Design review of the part built by this model. Coordinates are the model's own, in mm. A direction names the side the tool comes from. Round coordinates to 2 decimals unless told otherwise and drop trailing zeros. Order: outer loops, then holes, each group sorted by start corner. A loop starts at its lowest first (then second) coordinate and runs counter-clockwise, first axis right, second up. Notation, with made-up numbers: M -5.5,-30.5 L 22.5,-30.5 A32 ccw 22.5,-0.5 Z; hole C 11,-6 d4. An arc over 180 degrees is marked long. Write item = value, one per line. Start each with the question number.
```python
from build123d import *

# Parameters (mm, degrees)
SKETCH1_R     = 17.5
BODY_DEPTH    = 85
SKETCH2_W     = 1.5
SKETCH2_H     = 1.4
CHAMFER1_SIZE = 1


with BuildPart() as part:
    # Sketch1 → Body (new body)
    with BuildSketch(Plane.XY):
        Circle(SKETCH1_R)
    extrude(amount=BODY_DEPTH)

    # Sketch2 → Ret Ring Grooves (revolve, cut)
    with BuildSketch(Plane(origin=(0, 0, 0), x_dir=(0, 0, -1), z_dir=(1, 0, 0)), mode=Mode.PRIVATE) as ret_ring_grooves_sk:
        with Locations((-3.75, 16.8)):
            Rectangle(SKETCH2_W, SKETCH2_H)
        with Locations((-23.25, 16.8)):
            Rectangle(SKETCH2_W, SKETCH2_H)
        with Locations((-25.75, 16.8)):
            Rectangle(SKETCH2_W, SKETCH2_H)
        with Locations((-81.25, 16.8)):
            Rectangle(SKETCH2_W, SKETCH2_H)
    revolve(ret_ring_grooves_sk.sketch.rotate(Axis((0, 0, 85), (0, 0, -1)), 90), axis=Axis((0, 0, 85), (0, 0, -1)), mode=Mode.SUBTRACT)

    # Chamfer1
    chamfer1_edges = [part.edges().sort_by_distance(p)[0] for p in [
        (-17.5, 0, 0),
        (-17.5, 0, 85),
    ]]
    chamfer(chamfer1_edges, length=CHAMFER1_SIZE)


solid = part.part
```
(1) For faces 4 (the face through (15.357, -4.836, 3.74)), 5 (the face through (-13.887, -10.648, 53.122)), list the 3-axis set-ups (+Z, -Z, +X, -X, +Y, -Y) from which the entire face can be reached by the end or side of a thin tool; tool diameter is ignored.
(2) Insertion check: pin 1 (1 mm diameter, centred on x = 8, z = 40.5, fed in from +Y); pin 2 (1 mm diameter, centred on x = 3, z = 30.5, fed in from +Y); pin 3 (10 mm diameter, centred on y = 9, z = 46.5, fed in from -X). Each pin has a flat end and moves straight along its axis. Give the tip position at first contact, or say it passes through.
(3) For line 1 along Y through (x, z) = (-0.5, 5); line 2 along Z through (x, y) = (-15, 8.5), list the stretches that pass through material, from the lowest coordinate up. Write a range as [from, to].
(4) Draft analysis for pull direction Z (two halves, no side actions). For faces 1 (the face through (-15.5, 5.1, 82)), 2 (the face through (-13.887, -10.648, 24.493)), 3 (the face through (0, 0, 0)), state which applies: pulls with the +Z half, pulls with the -Z half, needs draft (parallel to the pull), parting line crosses it, or undercut.
(5) Consider section A-A, the plane z = 69. Write out the cut boundary in (x, y).
Completed:
q1.face_4 = none
q1.face_5 = +Z, -Z
q2.pin_1 = 15.81
q2.pin_2 = 17.32
q2.pin_3 = -17.04
q3.line_1 = [-17.49, 17.49]
q3.line_2 = [0.74, 3], [4.5, 22.5], [24, 25], [26.5, 80.5], [82, 84.26]
q4.face_1 = undercut
q4.face_2 = needs draft
q4.face_3 = pulls with the -Z half
q5.outline = C 0,0 d35
